Can you work these out from the drawing? Everything is in mm from the part's minimum corner. A direction names the side the tool comes from. Give positions to 0.01 mm unless a question says otherwise; leave off trailing zeros. Write each loop counter-clockwise with the first axis right and the second up, starting at its lowest first coordinate (ties: lowest second). Pieces come first, ordered by that corner, then holes. Notation, with made-up numbers: M -1,64.5 L 7,64.5 A18 ccw 7,92.5 Z; hole C 30.5,-1 d4. An arc over 180 degrees is marked long. One line per item, written item: value.
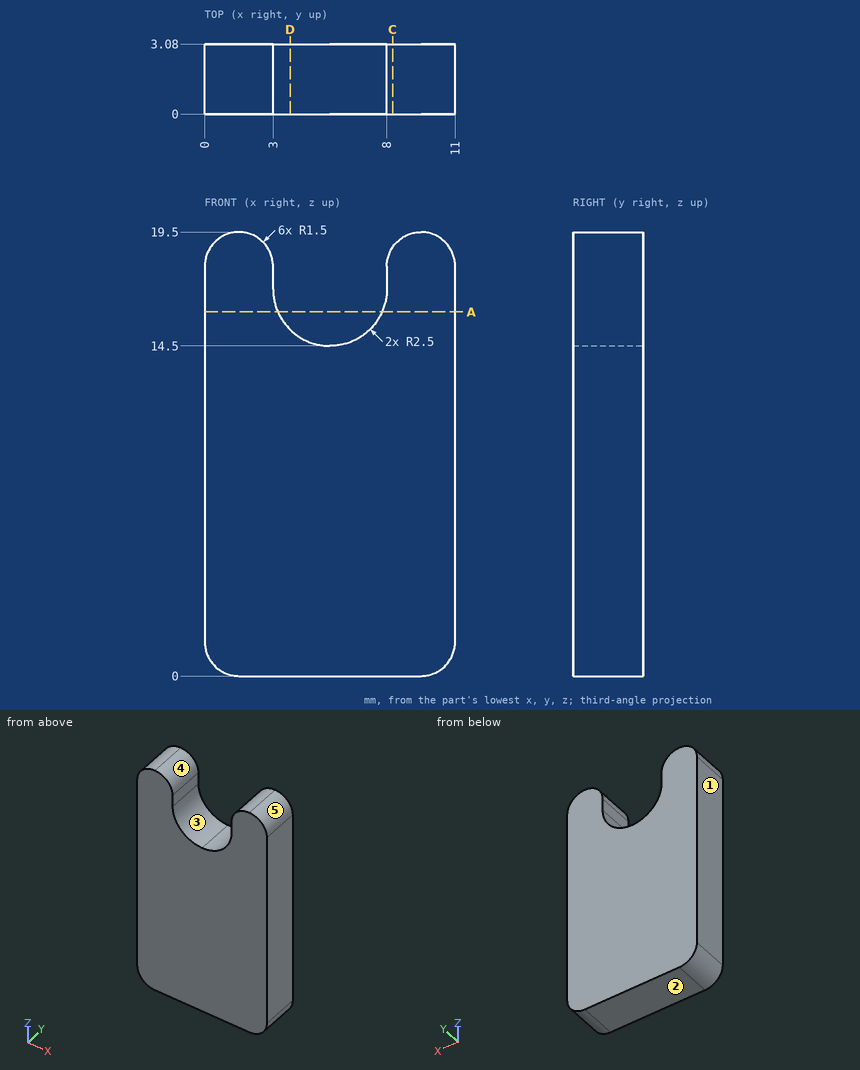
1) If we section it at C-C, the plane x = 8.25: Write out the boundary of the cut face in (y, z).
Outcome:
outline: M 0,0 L 3.08,0 L 3.08,18.83 L 0,18.83 Z
2) We'd pull the mould along X, two halves only. Please class the marked faces 1, 2 and 3: pulls with the +X half, pulls with the -X half, needs draft (parallel to the pull), parting line crosses it, or undercut.
Outcome:
face 1: pulls with the -X half
face 2: needs draft
face 3: undercut
3) On a 3-axis mill with a long thin cutter (end or side, diameter ignored), from which of +Z, -Z, +X, -X, +Y, -Y can I reach the whole of each face in a straight line? I mean the marked faces 4 and 5. Say none if no direction works.
Outcome:
face 4: +Z, +Y, -Y
face 5: +Z, +X, +Y, -Y
4) Please list where these lines run through material, in increasing order: L1, parallel to X at y = 2, z = 18.75; L2, parallel to X at y = 1.9, z = 16.25 (3 decimals); L3, parallel to Z at x = 2.25, y = 2.7. Write a range as from..to.
Outcome:
L1: x = 0.2..2.8, 8.2..10.8
L2: x = 0..3.115, 7.885..11
L3: z = 0..19.3
5) If we section it at A-A, the plane z = 16: Write out the boundary of the cut face in (x, y), then the cut area to 3 significant figures.
Outcome:
outline: M 0,0 L 3.21,0 L 3.21,3.08 L 0,3.08 Z; M 7.79,0 L 11,0 L 11,3.08 L 7.79,3.08 Z
area: 19.8 mm^2
6) I'm going to push flat-ended pins straight in: pin 1 (1 mm diameter, centred on x = 4, y = 1.5, fed in from +Z); pin 2 (1.1 mm diameter, centred on y = 1.5, z = 17.5, fed in from -X). Where does each tip first touch, or does it pass through?
Outcome:
pin 1: stops at z = 15.5
pin 2: stops at x = 0
7) If we section it at D-D, the plane x = 3.75: Write out the boundary of the cut face in (y, z).
Outcome:
outline: M 0,0 L 3.08,0 L 3.08,15.21 L 0,15.21 Z
